For this review, take the finished solid that the model builds, in its own axes (mm). Face numbers are marked on the shaded views. A direction names the side the tool comes from. Round coordinates to 2 decimals unless told otherwise and drop trailing zeros. Loops run counter-clockwise (first coordinate to the right, second up) from the corner with the lowest first, then second, coordinate; pieces in that order, holes last.
1) Take a section at A-A (y = 15.06). State the section outline as (x, z) points (3 decimals), then the cut area to 4 significant figures.
2) Mouldability with a two-part tool opening along Z and no side actions: class the marked faces 6, 7, 8 and 9 as pulls with the +Z half, pulls with the -Z half, needs draft (parallel to the pull), parting line crosses it, or undercut.
3) Insertion check: pin 1 (5 mm diameter, centred on x = 1, z = -18.5, fed in from -Y); pin 2 (1 mm diameter, centred on x = 20, z = -26.5, fed in from -Y); pin 3 (4.5 mm diameter, centred on y = 23.56, z = -15, fed in from +X); pin 4 (8 mm diameter, centred on x = 25.5, y = -10, fed in from +Z) (3 decimals). Each pin has a flat end and moves straight along its axis. Give the tip position at first contact, or say it passes through.
4) Take a section at B-B (z = -15). Give the number of separate pieces and of enclosed holes in the cut face, then the cut area to 3 significant figures.
5) Wall thickness on L1, parallel to X at y = 80.5, z = -25.25; L2, parallel to X at y = 17, z = -6.5; L3, parallel to Y at x = 22.75, z = -15 (3 decimals): over which ranges is each line inside the solid? List them lowest first.
6) Tool access review of the marked faces 1, 2, 3, 4 and 5: name each direction out of +Z, -Z, +X, -X, +Y, -Y from which nothing blocks a thin tool from reaching the whole face with its end or side.
7) Take a section at C-C (x = 27.5). State the section outline as (y, z) points (3 decimals), then the cut area to 3 significant figures.
8) Take a section at D-D (y = 62). State the section outline as (x, z) points, then the cut area to 3 significant figures.
Autodesk Inventor part; units mm, degrees
ref_plane "YZ Plane" through (0, 0, 0) normal (1, 0, 0) x (0, 1, 0)
ref_plane "XZ Plane" through (0, 0, 0) normal (0, 1, 0) x (-1, 0, 0)
ref_plane "XY Plane" through (0, 0, 0) normal (0, 0, 1) x (1, 0, 0)
sketch "Sketch1" plane through (0, 0, 0) normal (0, 0, 1) x (1, 0, 0)
  line L0 (0, 0) -> (25, 0)
  line L1 (25, 0) -> (25, 40)
  line L2 (25, 40) -> (0, 40)
  line L3 (0, 40) -> (0, 0)
  dimension "d1" = 25
  dimension "d2" = 40
  dimension "d3" = 25
extrude "Extrusion1" add sketch "Sketch1" against normal blind 30
sketch "Sketch2" plane through (25, 0, 0) normal (1, 0, 0) x (0, 0, -1)
  line L0 (0, 0) -> (30, 0)
  circle A0 centre (15, 6.56) radius 2.46
extrude "Extrusion2" cut sketch "Sketch2" against normal blind 30
sketch "Sketch3" plane through (0, 0, 0) normal (-1, 0, 0) x (0, 0, 1)
  line L0 (0, 0) -> (-30, 0)
  line L1 (-25.05, 0) -> (-4.95, 0)
  line L2 (-4.95, 0) -> (-4.95, 33.12)
  line L3 (-4.95, 33.12) -> (-25.05, 33.12)
  line L4 (-25.05, 33.12) -> (-25.05, 0)
  dimension "d11" = 20.1
extrude "Extrusion3" cut sketch "Sketch3" against normal blind 20
sketch "Sketch4" plane through (0, 0, 0) normal (0, -1, 0) x (1, 0, 0)
  line L0 (20, -4.95) -> (20, -25.05)
  line L1 (20, -15) -> (25, -15)
  line L2 (25, 0) -> (25, -30)
  line L3 (20, -8.025) -> (25, -8.025)
  line L4 (25, -8.025) -> (25, -21.975)
  line L5 (25, -21.975) -> (20, -21.975)
  line L6 (20, -21.975) -> (20, -8.025)
  line L7 (20, -8.025) -> (25, -21.975) construction
  line L8 (25, -8.025) -> (20, -21.975) construction
  line L9 (25, -12.54) -> (25, -17.46)
  point P0 (0, 0)
  point P1 (22.5, -15)
  dimension "d14" = 13.95
extrude "Extrusion4" add sketch "Sketch4" along normal blind 15
sketch "Sketch5" plane through (20, 0, 0) normal (-1, 0, 0) x (0, 0, 1)
  circle A0 centre (-15, 6.56) radius 2.46
  circle A1 centre (-15, 6.56) radius 4.7025
  circle A2 centre (-15, 6.56) radius 2.46
  circle A3 centre (-15, 6.56) radius 2.46
  point P0 (0, 0)
  dimension "d17" = 9.405
extrude "Extrusion5" cut sketch "Sketch5" against normal blind 2.1
sketch "Sketch6" plane through (25, 0, 0) normal (1, 0, 0) x (0, 0, -1)
  circle A0 centre (15, 6.56) radius 4.7025
  line L0 (15, 6.56) -> (15, 23.56)
  circle A1 centre (15, 23.56) radius 2.46
  point P0 (0, 0)
  dimension "d20" = 17
  dimension "d21" = 4.92
extrude "Extrusion6" cut sketch "Sketch6" against normal blind 10 contours A1
sketch "Sketch7" plane through (20, 0, 0) normal (-1, 0, 0) x (0, 0, 1)
  circle A0 centre (-15, 23.56) radius 2.46
  circle A1 centre (-15, 23.56) radius 4.7025
  point P0 (0, 0)
  dimension "d24" = 9.405
extrude "Extrusion7" cut sketch "Sketch7" against normal blind 2.1
sketch "Sketch9" plane through (25, 0, 0) normal (1, 0, 0) x (0, 0, -1)
  circle A0 centre (15, 6.56) radius 2.46
  circle A1 centre (15, 6.56) radius 2.46
  circle A2 centre (15, 23.56) radius 2.46
  circle A3 centre (15, 23.56) radius 2.46
  line L0 (30, 40) -> (30, 0)
  line L1 (30, 0) -> (30, 40)
  line L2 (30, 40) -> (0, 40)
  line L3 (0, 40) -> (0, 0)
  line L4 (0, 0) -> (8.025, 0)
  line L5 (21.975, 0) -> (21.975, -15)
  line L6 (21.975, -15) -> (8.025, -15)
  line L7 (8.025, -15) -> (8.025, 0)
  line L8 (0, 0) -> (8.025, 0)
  line L9 (21.975, 0) -> (30, 0)
extrude "Extrusion8" add sketch "Sketch9" along normal blind 5
sketch "Sketch10" plane through (0, 40, 0) normal (0, 1, 0) x (1, 0, 0)
  line L0 (0, 30) -> (30, 30)
  line L1 (30, 0) -> (0, 0)
  line L2 (0, 30) -> (30, 30)
  line L3 (30, 30) -> (30, 0)
  line L4 (30, 0) -> (0, 0)
  line L5 (0, 0) -> (0, 30)
extrude "Extrusion9" add sketch "Sketch10" along normal blind 30
sketch "Sketch12" plane through (30, 0, 0) normal (1, 0, 0) x (0, 0, -1)
  circle A0 centre (15, 6.56) radius 2.46
  line L0 (15, 6.56) -> (15, 15.06)
  circle A1 centre (15, 15.06) radius 2.525
  point P0 (0, 0)
  dimension "d31" = 8.5
  dimension "d33" = 5.05
extrude "Extrusion10" cut sketch "Sketch12" against normal blind 30 contours A1
sketch "Sketch14" plane through (0, 0, 0) normal (0, 0, 1) x (1, 0, 0)
  line L0 (30, 70) -> (0, 70)
  line L1 (0, 70) -> (0, 85)
  line L2 (-15, 100) -> (-23, 100)
  line L3 (30, 0) -> (30, 70)
  line L4 (30, 113) -> (30, 70)
  arc A0 (0, 85) -> (-15, 100) centre (-15, 85) ccw
  line L5 (30, 105) -> (30, 100)
  line L6 (-23, 128) -> (15, 128)
  line L7 (-19, 126) -> (-23, 128)
  line L8 (-19, 126) -> (-15, 114)
  line L9 (-19, 102) -> (-23, 100)
  line L10 (-19, 102) -> (-15, 114)
  line L11 (30, 113) -> (15, 128)
  point P0 (0, 0)
  point P1 (0, 100)
  dimension "d47" = 30
  dimension "d54" = 15
  dimension "d69" = 28
extrude "Extrusion12" add sketch "Sketch14" against normal blind 30
sketch "Sketch15" plane through (0, 0, -25.05) normal (-1, 0, 0) x (0, 0, 1)
  line L0 (0, 33.12) -> (20.1, 33.12)
  line L1 (20.1, 33.12) -> (20.1, 0)
  line L2 (0, 33.12) -> (20.1, 33.12)
  line L3 (20.1, 33.12) -> (20.1, 31.1)
  line L4 (20.1, 31.1) -> (0, 31.1)
  line L5 (0, 31.1) -> (0, 33.12)
  point P0 (25.05, 0)
  dimension "d57" = 2.02
extrude "Extrusion13" add sketch "Sketch15" against normal blind 20
properties part number "24mm_x_30mm"
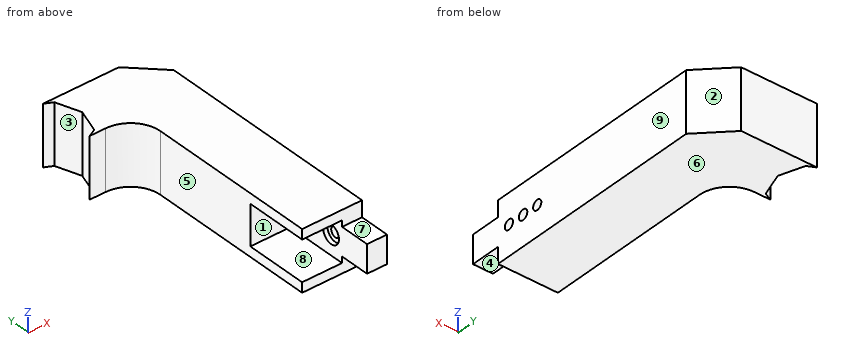
Response:
1. outline: (0, -30) - (30, -30) - (30, -17.525) - (20, -17.525) - (20, -25.05) - (0, -25.05) - close; (0, -4.95) - (20, -4.95) - (20, -12.475) - (30, -12.475) - (30, 0) - (0, 0) - close
1. area: 447.5 mm2
2. face 6: pulls with the -Z half
2. face 7: pulls with the +Z half
2. face 8: undercut
2. face 9: needs draft
3. pin 1: stops at y = 31.1
3. pin 2: stops at y = 0
3. pin 3: passes through
3. pin 4: stops at z = -8.025
4. separate pieces: 4
4. enclosed holes: 0
4. area: 3,630 mm2
5. L1: x = 0 to 30
5. L2: x = 20 to 30
5. L3: y = -15 to 4.1, 9.02 to 12.535, 17.585 to 21.1, 26.02 to 120.25
6. face 1: -X, -Y
6. face 2: +Z, -Z, +X, +Y
6. face 3: +Z, -Z, -X
6. face 4: -Z, +X, -X, -Y
6. face 5: +Z, -Z, -X, -Y
7. outline: (-15, -21.975) - (0, -21.975) - (0, -30) - (115.5, -30) - (115.5, 0) - (0, 0) - (0, -8.025) - (-15, -8.025) - close; hole circle Ø4.92 at (6.56, -15); hole circle Ø5.05 at (15.06, -15); hole circle Ø4.92 at (23.56, -15)
7. area: 3,620 mm2
8. outline: (0, -30) - (30, -30) - (30, 0) - (0, 0) - close
8. area: 900 mm2
